```python
from build123d import *

# Parameters (mm, degrees)
SKETCH1_R               = 27.686
SKETCH1_R_2             = 21.336
BOSS_EXTRUDE1_DEPTH     = 63.5
BOSS_EXTRUDE2_START     = -3.175
SKETCH2_R               = 34.036
SKETCH2_R_2             = 27.686
BOSS_EXTRUDE2_DEPTH     = 3.175
CUT_EXTRUDE1_DEPTH      = 101.6
CUT_EXTRUDE1_DEPTH_BACK = 101.6
SKETCH3_W               = 97.716171251
SKETCH3_H               = 43.59719505
SKETCH4_R               = 1.4732
CUT_EXTRUDE2_DEPTH      = 101.6
SKETCH5_W               = 45.490276776
SKETCH5_H               = 8.374778988
CUT_EXTRUDE3_DEPTH      = 101.6
SKETCH6_R               = 22.86
CUT_EXTRUDE4_DEPTH      = 14.478


with BuildPart() as part:
    # Sketch1 → Boss-Extrude1 (new body)
    with BuildSketch(Plane.XY):
        Circle(SKETCH1_R)
        Circle(SKETCH1_R_2, mode=Mode.SUBTRACT)
    extrude(amount=BOSS_EXTRUDE1_DEPTH)

    # Sketch2 → Boss-Extrude2 (add)
    with BuildSketch(Plane.XY.offset(63.5).offset(BOSS_EXTRUDE2_START)):
        Circle(SKETCH2_R)
        Circle(SKETCH2_R_2, mode=Mode.SUBTRACT)
    extrude(amount=BOSS_EXTRUDE2_DEPTH)

    # Sketch3 → Cut-Extrude1 (cut, two sides: drawn at the far end of the back side and taken through both)
    with BuildSketch(Plane(origin=(0, 0, 60.325), x_dir=(-1, 0, 0), z_dir=(0, 0, -1)).offset(-CUT_EXTRUDE1_DEPTH_BACK)):
        with Locations((3.507260384, 21.798597525)):
            Rectangle(SKETCH3_W, SKETCH3_H)
    extrude(amount=CUT_EXTRUDE1_DEPTH + CUT_EXTRUDE1_DEPTH_BACK, mode=Mode.SUBTRACT)

    # Sketch4 → Cut-Extrude2 (cut)
    with BuildSketch(Plane(origin=(0, 0, 60.325), x_dir=(-1, 0, 0), z_dir=(0, 0, -1))):
        with Locations((-30.183908954, -5.789782512)):
            Circle(SKETCH4_R)
        with Locations((30.183908954, -5.789782512)):
            Circle(SKETCH4_R)
        with Locations((-20.137167932, -23.218191337)):
            Circle(SKETCH4_R)
        with Locations((20.137167932, -23.218191337)):
            Circle(SKETCH4_R)
        with Locations((0, -30.734181969)):
            Circle(SKETCH4_R)
    extrude(amount=-CUT_EXTRUDE2_DEPTH, mode=Mode.SUBTRACT)

    # Sketch5 → Cut-Extrude3 (cut)
    with BuildSketch(Plane(origin=(0, 0, 60.325), x_dir=(-1, 0, 0), z_dir=(0, 0, -1))):
        with Locations((-0.190335886, -32.086257649)):
            Rectangle(SKETCH5_W, SKETCH5_H)
    extrude(amount=-CUT_EXTRUDE3_DEPTH, mode=Mode.SUBTRACT)

    # Sketch6 → Cut-Extrude4 (cut)
    with BuildSketch(Plane(origin=(0, 0, 0), x_dir=(-1, 0, 0), z_dir=(0, 0, -1))):
        Circle(SKETCH6_R)
    extrude(amount=-CUT_EXTRUDE4_DEPTH, mode=Mode.SUBTRACT)


solid = part.part
```
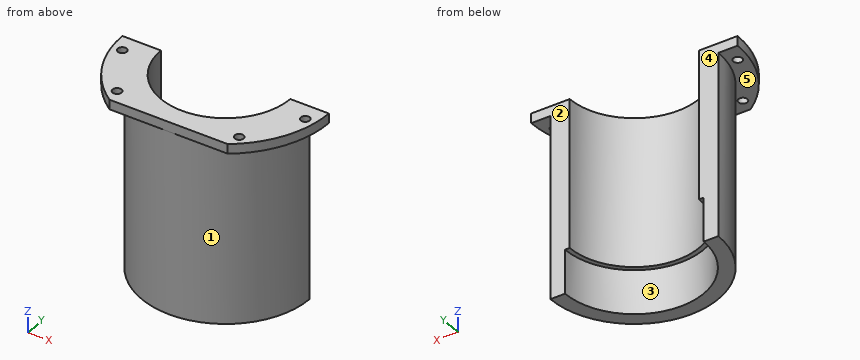
Input: part model. Units: mm. Frame: model coordinates. Face numbers are marked on the shaded views. A direction names the side the tool comes from. Coordinates: 2 decimals unless noted, no trailing zeros. Loops run counter-clockwise (first coordinate to the right, second up) from the corner with the lowest first, then second, coordinate; pieces in that order, holes last. Notation, with made-up numbers: (23, -36) -> (66, -36) arc R26 cw to (66, -7) -> close; hole circle Ø2 at (66, 60.5). An arc over 180 degrees is marked (long way). Use a Markdown table: item, result.
1) Cut plane A-A (x = 0). Return the cut outline in (y, z) (3 decimals), then the cut area to 3 significant figures.
Results found:
| item | result |
|---|---|
| outline | (-27.899, 60.325) -> (-27.686, 60.325) -> (-27.686, 0) -> (-22.86, 0) -> (-22.86, 14.478) -> (-21.336, 14.478) -> (-21.336, 63.5) -> (-27.899, 63.5) -> close |
| area | 382 mm2 |
2) Pull-direction query (X, two-part tool) for the marked faces 1, 2 and 3; classes: released by +X, released by -X, zero draft, split by the parting line, or undercut.
Results found:
| item | result |
|---|---|
| face 1 | split by the parting line |
| face 2 | zero draft |
| face 3 | undercut |
3) Material intervals for line 1 along Z through (x, y) = (-8, -20.75); line 2 along Z through (x, y) = (-18, -22.5) (3 decimals); line 3 along X through (y, z) = (-18, 56), sorted ascending. Write a range as from..to.
Results found:
| item | result |
|---|---|
| line 1 | z = 14.48..63.5 |
| line 2 | z = 60.325..63.5 |
| line 3 | x = -21.04..-11.46, 11.46..21.04 |
4) Contact query for flat-ended pins moving along their axis: pin 1 (4.5 mm diameter, centred on x = -20.14, y = -23.22, fed in from -Z) (3 decimals); pin 2 (4 mm diameter, centred on x = -10, z = 53.5, fed in from -Y) (3 decimals); pin 3 (1.8 mm diameter, centred on x = -30.18, y = -5.79, fed in from -Z); pin 4 (1 mm diameter, centred on y = -24.5, z = 35.5, fed in from +X). Output: stop coordinate, or through.
Results found:
| item | result |
|---|---|
| pin 1 | stops at z = 60.325 |
| pin 2 | stops at y = -26.505 |
| pin 3 | passes through |
| pin 4 | stops at x = 13.8 |
5) Access query for the marked faces 4 and 5. Directions: +Z, -Z, +X, -X, +Y, -Y. A direction counts if a zero-diameter tool reaches every point of the face in a straight line with its end or side. Return the directions, or none.
Results found:
| item | result |
|---|---|
| face 4 | +Z, -Z, +X, -X, +Y |
| face 5 | -Z, -Y |
6) Cut plane C-C (x = 20.5). Return the cut outline in (y, z) (3 decimals).
Results found:
| item | result |
|---|---|
| outline | (-27.17, 60.325) -> (-24.646, 60.325) -> (-24.646, 63.5) -> (-27.17, 63.5) -> close; (-21.79, 60.325) -> (-18.608, 60.325) -> (-18.608, 0) -> (-10.116, 0) -> (-10.116, 14.478) -> (-5.914, 14.478) -> (-5.914, 63.5) -> (-21.79, 63.5) -> close |
7) Cut plane B-B (z = 29.5). Return the cut outline in (x, y), then the cut area to 3 significant figures.
Results found:
| item | result |
|---|---|
| outline | (-27.69, 0) arc R27.69 ccw to (27.69, 0) -> (21.34, 0) arc R21.34 cw to (-21.34, 0) -> close |
| area | 489 mm2 |
